Geometry check sheet. Reference: the model listing, model coordinates, mm. A direction names the side the tool comes from. Round coordinates to 2 decimals unless told otherwise and drop trailing zeros. Write each loop counter-clockwise with the first axis right and the second up, starting at its lowest first coordinate (ties: lowest second). Pieces come first, ordered by that corner, then holes.
Item 1: Scan lines: probe 1 along X at (y, z) = (66, 13); probe 2 along X at (y, z) = (-12.5, 42); probe 3 along Y at (x, z) = (-66.5, 40). Record each from-to range of solid material in increasing order.
Item 2: Cross-section at A-A (y = 0). Enter the section's corners in (x, z), then the cut area to 3 significant figures.
Item 3: Draft check along X on faces 1 (the face through (100.15, 31.54, 24.65)), 2 (the face through (-1, -1, 50)), 3 (the face through (66.144, -1, 25)). Enter one of: pulls with the +X half, pulls with the -X half, needs draft (parallel to the pull), parting line crosses it, or undercut.
Item 4: Cross-section at C-C (x = -87). Enter the section's corners in (y, z), then the cut area to 3 significant figures.
Item 5: Depth check by flat-ended pin: P1, Ø1.5, axis at x = -83, z = 38.5, coming from the +Y side; P2, Ø15, axis at y = -10.5, z = 35, coming from the -X side; P3, Ø6, axis at x = 14.5, z = 41.5, coming from the -Y side. Enter the tip coordinate at first touch or a pass-through.
Item 6: Cross-section at B-B (z = 18). Enter the section's corners in (x, y), then the cut area to 3 significant figures.
Item 7: Cross-section at D-D (y = 45.5). Enter the section's corners in (x, z).
Item 8: Access from +Z, -Z, +X, -X, +Y, -Y to the whole of each face (thin tool, end or side, straight path). Record for faces 4 (the face through (-66.144, -1, 25)), 5 (the face through (-1, -1, 0)).
from build123d import *

# Parameters (mm, degrees)
F0_R      = 105
F0_R_2    = 100
F1_DEPTH  = 50
F3_W      = 132.2875655532
F3_H      = 50
F4_FACE_W = 132.2875655532
F4_FACE_H = 50


with BuildPart() as f1:
    # F0 (on Top) → F1 (new body)
    with BuildSketch(Plane.XY):
        Circle(F0_R)
        Circle(F0_R_2, mode=Mode.SUBTRACT)
    extrude(amount=F1_DEPTH)

    # F3 (on offset) → F4 (join, up to the next surface of F1)
    with BuildSketch(Plane.XZ.offset(75)):
        with Locations((0, 25)):
            Rectangle(F3_W, F3_H)
    extrude(until=Until.NEXT)

    # F4_face (on face) → F5 (join, up to the next surface of F1)
    with BuildSketch(Plane(origin=(0, -75, 25), x_dir=(1, 0, 0), z_dir=(0, 1, 0))):
        Rectangle(F4_FACE_W, F4_FACE_H)
    extrude(until=Until.NEXT)


solid = f1.part
Resolved:
1. probe 1: x = -81.66 to -75.13, -66.14 to 66.14, 75.13 to 81.66
1. probe 2: x = -104.25 to -99.22, -66.14 to 66.14, 99.22 to 104.25
1. probe 3: y = -81.26 to -74.68, 74.68 to 81.26
2. outline: (-105, 0) - (-100, 0) - (-100, 50) - (-105, 50) - close; (-66.14, 0) - (66.14, 0) - (66.14, 50) - (-66.14, 50) - close; (100, 0) - (105, 0) - (105, 50) - (100, 50) - close
2. area: 7,110 mm2
3. face 1: parting line crosses it
3. face 2: needs draft
3. face 3: undercut
4. outline: (-58.79, 0) - (-49.31, 0) - (-49.31, 50) - (-58.79, 50) - close; (49.31, 0) - (58.79, 0) - (58.79, 50) - (49.31, 50) - close
4. area: 948 mm2
5. P1: stops at y = 65.27
5. P2: stops at x = -104.96
5. P3: stops at y = -104.37
6. outline: circle Ø210 at (0, 0); hole (-66.14, -75) - (-66.14, 75) arc R100 ccw to start; hole (66.14, -75) arc R100 ccw to (66.14, 75) - close
6. area: 27,600 mm2
7. outline: (-94.63, 0) - (-89.05, 0) - (-89.05, 50) - (-94.63, 50) - close; (-66.14, 0) - (66.14, 0) - (66.14, 50) - (-66.14, 50) - close; (89.05, 0) - (94.63, 0) - (94.63, 50) - (89.05, 50) - close
8. face 4: +Z, -Z
8. face 5: -Z, +X, -X, +Y, -Y
